Model file for the job. Use its own axes, mm. Coordinates: 2 decimals unless noted, no trailing zeros. Order: outer loops, then holes, each group sorted by start corner. A loop starts at its lowest first (then second) coordinate and runs counter-clockwise, first axis right, second up. Notation, with made-up numbers: (21, 77.5) -> (28, 77.5) arc R13 cw to (28, 87.5) -> close; hole circle Ø7 at (-35, 28). An arc over 180 degrees is marked (long way). Return JSON: item names as keys, results as strings. Group by question number.
1) Cut at C-C (z = 4.05). Write the cut outline in (x, y) (3 decimals).
2) Cut at B-B (x = 719.5). Write the cut outline in (y, z), and give its area (3 significant figures).
3) Cut at A-A (y = 85.5). Write the cut outline in (x, z), and give its area (3 significant figures).
4) Cut at D-D (x = 504). Write the cut outline in (y, z).
5) Probe line 1 (Y direction, x = 464, z = 1.65); line 2 (X direction, y = 367.5, z = 1.95); line 3 (Y direction, x = 619, z = 0.75). List the from-to ranges inside material, lowest first.
Autodesk Inventor part; units mm, degrees
ref_plane "YZ Plane" through (0, 0, 0) normal (1, 0, 0) x (0, 1, 0)
ref_plane "XZ Plane" through (0, 0, 0) normal (0, 1, 0) x (-1, 0, 0)
ref_plane "XY Plane" through (0, 0, 0) normal (0, 0, 1) x (1, 0, 0)
sketch "Sketch1" plane through (0, 0, 0) normal (0, 0, 1) x (1, 0, 0)
  line L0 (0, 0) -> (1117.6, 0)
  line L1 (1117.6, 0) -> (1117.6, 800.1)
  line L2 (1117.6, 800.1) -> (0, 800.1)
  line L3 (0, 800.1) -> (0, 0)
  line L4 (50.8, 749.3) -> (1066.8, 749.3)
  line L5 (1066.8, 749.3) -> (1066.8, 50.8)
  line L6 (1066.8, 50.8) -> (50.8, 50.8)
  line L7 (50.8, 50.8) -> (50.8, 749.3)
  dimension "d0" = 800.1
  dimension "d1" = 1117.6
  dimension "d2" = 50.8
extrude "Extrusion1" add sketch "Sketch1" along normal blind 4.7752
sketch "Sketch2" plane through (0, 0, 4.7752) normal (0, 0, 1) x (1, 0, 0)
  line L0 (1066.8, 50.8) -> (50.8, 50.8)
  line L1 (0, 0) -> (0, 800.1)
  line L2 (1117.6, 0) -> (0, 0)
  line L3 (492.125, 0) -> (625.475, 0)
  line L4 (625.475, 0) -> (625.475, 50.8)
  line L5 (625.475, 50.8) -> (492.125, 50.8)
  line L6 (492.125, 50.8) -> (492.125, 0)
  dimension "d5" = 133.35
  dimension "d6" = 492.125
extrude "Extrusion2" cut sketch "Sketch2" against normal through all
properties part number "backboardtape"
Answers below:
{
 "1": {"outline": "(0, 0) -> (492.125, 0) -> (492.125, 50.8) -> (50.8, 50.8) -> (50.8, 749.3) -> (1066.8, 749.3) -> (1066.8, 50.8) -> (625.475, 50.8) -> (625.475, 0) -> (1117.6, 0) -> (1117.6, 800.1) -> (0, 800.1) -> close"},
 "2": {"outline": "(0, 0) -> (50.8, 0) -> (50.8, 4.78) -> (0, 4.78) -> close; (749.3, 0) -> (800.1, 0) -> (800.1, 4.78) -> (749.3, 4.78) -> close", "area": "485 mm^2"},
 "3": {"outline": "(0, 0) -> (50.8, 0) -> (50.8, 4.78) -> (0, 4.78) -> close; (1066.8, 0) -> (1117.6, 0) -> (1117.6, 4.78) -> (1066.8, 4.78) -> close", "area": "485 mm^2"},
 "4": {"outline": "(749.3, 0) -> (800.1, 0) -> (800.1, 4.78) -> (749.3, 4.78) -> close"},
 "5": {"line 1": "y = 0 to 50.8, 749.3 to 800.1", "line 2": "x = 0 to 50.8, 1066.8 to 1117.6", "line 3": "y = 749.3 to 800.1"}
}
